```python
from build123d import *

# Parameters (mm, degrees)
F0_R     = 90
F0_R_2   = 75
F1_DEPTH = 20


with BuildPart() as f1:
    # F0 (on Top) → F1 (new body)
    with BuildSketch(Plane.XY):
        Circle(F0_R)
        Circle(F0_R_2, mode=Mode.SUBTRACT)
    extrude(amount=F1_DEPTH)

    # F2 (on face) → F3 (revolve)
    with BuildSketch(Plane.XY.offset(20)):
        with BuildLine():
            Line((-75.3442101292, -43.5), (-66.6839560914, -38.5))
            ThreePointArc((-66.6839560914, -38.5), (-73.5140831103, -36.6698729811), (-75.3442101292, -43.5))
        make_face()
    revolve(axis=Axis((-77.9422863406, -45, 20), (0.8660254038, 0.5, 0)))

    # F4 (on face) → F5 (revolve)
    with BuildSketch(Plane.XY.offset(20)):
        with BuildLine():
            Line((66.6839560914, -38.5), (75.3442101292, -43.5))
            ThreePointArc((75.3442101292, -43.5), (73.5140831103, -36.6698729811), (66.6839560914, -38.5))
        make_face()
    revolve(axis=Axis((77.9422863406, -45, 20), (-0.8660254038, 0.5, 0)))

    # F6 (on face) → F7 (revolve)
    with BuildSketch(Plane.XY.offset(20)):
        with BuildLine():
            Line((0, 77), (0, 87))
            ThreePointArc((0, 87), (-5, 82), (0, 77))
        make_face()
    revolve(axis=Axis((0, 90, 20), (0, -1, 0)))


solid = f1.part
```
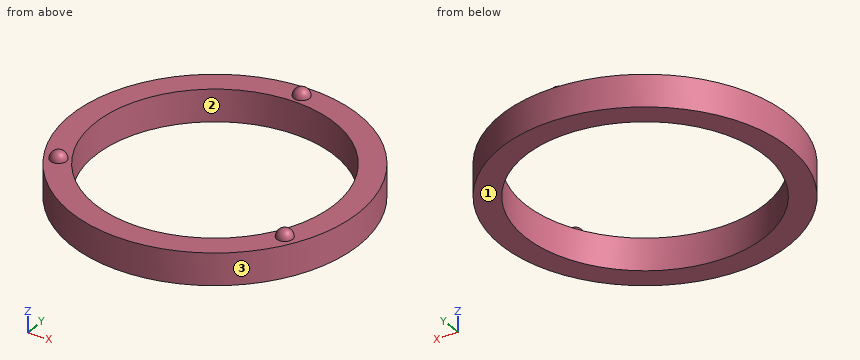
Input: part model. Units: mm. Frame: model coordinates. Face numbers are marked on the shaded views. Round coordinates to 2 decimals unless told otherwise and drop trailing zeros. Order: outer loops, then holes, each group sorted by start corner. A loop starts at its lowest first (then second) coordinate and runs counter-clockwise, first axis right, second up. Notation, with made-up numbers: (-18.75, 32) - (3.25, 32) arc R20 ccw to (3.25, 47) - close; hole circle Ø3 at (24.25, 2.5). An arc over 180 degrees is marked (long way). Answer in a Markdown table with one row per item.
Item 1: Section query B-B (x = 0). Return the cut outline in (y, z).
Model answer:
| item | result |
|---|---|
| outline | (-90, 0) - (-75, 0) - (-75, 20) - (-90, 20) - close; (75, 0) - (90, 0) - (90, 20) - (87, 20) arc R5 ccw to (77, 20) - (75, 20) - close |
Item 2: Section query D-D (y = -51). Return the cut outline in (x, z).
Model answer:
| item | result |
|---|---|
| outline | (-74.16, 0) - (-54.99, 0) - (-54.99, 20) - (-74.16, 20) - close; (54.99, 0) - (74.16, 0) - (74.16, 20) - (54.99, 20) - close |
Item 3: Line query: line 1 (Y direction, x = 0, z = 6); line 2 (X direction, y = 68.5, z = 8); line 3 (Z direction, x = -65, y = 44). Output: solid intervals per line, ascending.
Model answer:
| item | result |
|---|---|
| line 1 | y = -90 to -75, 75 to 90 |
| line 2 | x = -58.38 to -30.54, 30.54 to 58.38 |
| line 3 | z = 0 to 20 |
Item 4: Mould query, pull axis X, two halves, no side actions, for the marked faces 1, 2 and 3. Classes: released by +X, released by -X, zero draft, split by the parting line, or undercut.
Model answer:
| item | result |
|---|---|
| face 1 | zero draft |
| face 2 | undercut |
| face 3 | split by the parting line |
Item 5: Section query A-A (y = 0). Return the cut outline in (x, z).
Model answer:
| item | result |
|---|---|
| outline | (-90, 0) - (-75, 0) - (-75, 20) - (-90, 20) - close; (75, 0) - (90, 0) - (90, 20) - (75, 20) - close |
Item 6: Section query C-C (z = 16). Return the cut outline in (x, y), then the cut area to 3 significant figures.
Model answer:
| item | result |
|---|---|
| outline | circle Ø180 at (0, 0); hole circle Ø150 at (0, 0) |
| area | 7,780 mm² |
Item 7: Pin query (flat end, axial travel): pin 1 (2 mm diameter, centred on y = -8.5, z = 16.5, fed in from +X); pin 2 (6 mm diameter, centred on y = 54, z = 7, fed in from +X); pin 3 (5 mm diameter, centred on x = 59, z = 20, fed in from +Y). Return the tip coordinate at first contact, or that it passes through.
Model answer:
| item | result |
|---|---|
| pin 1 | stops at x = 89.69 |
| pin 2 | stops at x = 74.16 |
| pin 3 | stops at y = 70.06 |
